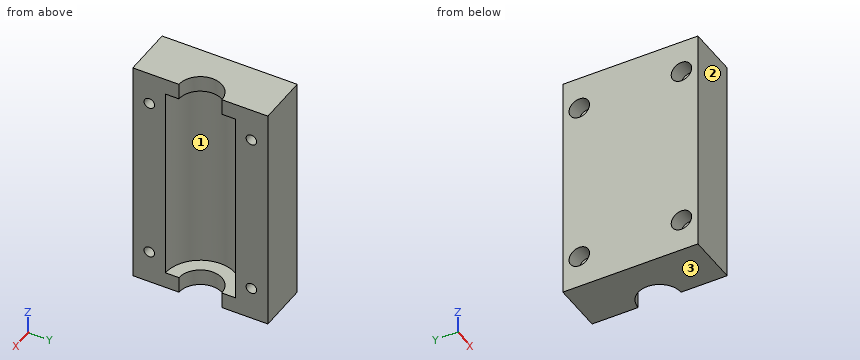
from build123d import *

# Parameters (mm, degrees)
PAD_DEPTH       = 35
SKETCH001_R     = 10.6
POCKET_DEPTH    = 30.1
SKETCH002_R     = 1.6
POCKET001_DEPTH = 15.501
SKETCH003_R     = 3.1
POCKET002_DEPTH = 5


with BuildPart() as part:
    # Sketch → Pad (new body, symmetric)
    with BuildSketch(Plane.XY):
        with BuildLine():
            ThreePointArc((0, 6.5), (-6.5, 0), (0, -6.5))
            Line((0, -20.5), (0, -6.5))
            Line((-15.5, -20.5), (0, -20.5))
            Line((-15.5, 20.5), (-15.5, -20.5))
            Line((0, 20.5), (-15.5, 20.5))
            Line((0, 6.5), (0, 20.5))
        make_face()
    extrude(amount=PAD_DEPTH, both=True)

    # Sketch001 → Pocket (cut, symmetric)
    with BuildSketch(Plane.XY):
        Circle(SKETCH001_R)
    extrude(amount=POCKET_DEPTH, both=True, mode=Mode.SUBTRACT)

    # Sketch002 → Pocket001 (cut, through all)
    with BuildSketch(Plane.YZ):
        with Locations((-15.5, 25)):
            Circle(SKETCH002_R)
        with Locations((-15.5, -25)):
            Circle(SKETCH002_R)
        with Locations((15.5, 25)):
            Circle(SKETCH002_R)
        with Locations((15.5, -25)):
            Circle(SKETCH002_R)
    extrude(amount=-POCKET001_DEPTH, mode=Mode.SUBTRACT)

    # Sketch003 (on Face7 of Pocket001) → Pocket002 (cut)
    with BuildSketch(Plane(origin=(-15.5, 0, 0), x_dir=(0, -1, 0), z_dir=(-1, 0, 0))):
        with Locations((-15.5, 25)):
            Circle(SKETCH003_R)
        with Locations((15.5, 25)):
            Circle(SKETCH003_R)
        with Locations((15.5, -25)):
            Circle(SKETCH003_R)
        with Locations((-15.5, -25)):
            Circle(SKETCH003_R)
    extrude(amount=-POCKET002_DEPTH, mode=Mode.SUBTRACT)


solid = part.part
Can you work these out from the model? Positions are in its coordinate system, mm. Face numbers are marked on the shaded views. Coordinates: 2 decimals unless noted, no trailing zeros. Order: outer loops, then holes, each group sorted by start corner. A loop starts at its lowest first (then second) coordinate and runs counter-clockwise, first axis right, second up. Notation, with made-up numbers: M -6.75,-19 L 3.25,-19 A11 cw 3.25,-14 Z; hole C -9.5,-3 d1. An arc over 180 degrees is marked long. Answer as CSV lines item,"result".
(1) Suppose I cut it at C-C on z = 25. Please give me the cut outline in (x, y).
Geometry check:
outline,"M -15.5,-20.5 L 0,-20.5 L 0,-17.1 L -10.5,-17.1 L -10.5,-18.6 L -15.5,-18.6 Z; M -15.5,-12.4 L -10.5,-12.4 L -10.5,-13.9 L 0,-13.9 L 0,-10.6 A10.6 cw 0,10.6 L 0,13.9 L -10.5,13.9 L -10.5,12.4 L -15.5,12.4 Z; M -15.5,18.6 L -10.5,18.6 L -10.5,17.1 L 0,17.1 L 0,20.5 L -15.5,20.5 Z"
(2) Suppose I cut it at B-B on x = -9. Please give me the cut outline in (y, z), plus the area to 3 significant figures.
Geometry check:
outline,"M -20.5,-35 L 20.5,-35 L 20.5,35 L -20.5,35 Z; hole C -15.5,-25 d3.2; hole C -15.5,25 d3.2; hole M -5.6,-30.1 L 5.6,-30.1 L 5.6,30.1 L -5.6,30.1 Z; hole C 15.5,-25 d3.2; hole C 15.5,25 d3.2"
area,"2,160 mm^2"
(3) Suppose I cut it at D-D on y = 0. Please give me the cut outline in (x, z), plus the area to 3 significant figures.
Geometry check:
outline,"M -15.5,-35 L -6.5,-35 L -6.5,-30.1 L -10.6,-30.1 L -10.6,30.1 L -6.5,30.1 L -6.5,35 L -15.5,35 Z"
area,"383 mm^2"
(4) If we mould it in two halves opening along Z, with no side actions, what happens to the marked faces 1, 2 and 3? For each: released by +Z, released by -Z, zero draft, split by the parting line, or undercut.
Geometry check:
face 1,"undercut"
face 2,"zero draft"
face 3,"released by -Z"
(5) Suppose I cut it at A-A on y = 15.5. Please give me the cut outline in (x, z).
Geometry check:
outline,"M -15.5,-35 L 0,-35 L 0,-26.6 L -10.5,-26.6 L -10.5,-28.1 L -15.5,-28.1 Z; M -15.5,-21.9 L -10.5,-21.9 L -10.5,-23.4 L 0,-23.4 L 0,23.4 L -10.5,23.4 L -10.5,21.9 L -15.5,21.9 Z; M -15.5,28.1 L -10.5,28.1 L -10.5,26.6 L 0,26.6 L 0,35 L -15.5,35 Z"
(6) Please list where these lines run through material, in increasing order: L1, parallel to Z at x = -5, y = -15.5; L2, parallel to Z at x = -11.75, y = -15.5; L3, parallel to Z at x = -4, y = 7.5.
Geometry check:
L1,"-35 to -26.6, -23.4 to 23.4, 26.6 to 35"
L2,"-35 to -28.1, -21.9 to 21.9, 28.1 to 35"
L3,"-35 to -30.1, 30.1 to 35"
(7) I'm going to push flat-ended pins straight in: pin 1 (6 mm diameter, centred on x = -5, y = 2.5, fed in from -Z); pin 2 (4 mm diameter, centred on y = -15.5, z = -25, fed in from -X). Where does each tip first touch, or does it pass through?
Geometry check:
pin 1,"z = -35"
pin 2,"x = -10.5"
